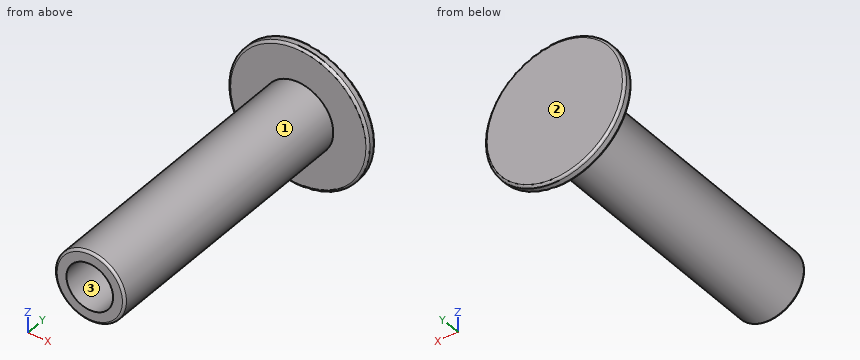
Autodesk Inventor part; units mm, degrees
ref_plane "YZ Plane" through (0, 0, 0) normal (1, 0, 0) x (0, 1, 0)
ref_plane "XZ Plane" through (0, 0, 0) normal (0, 1, 0) x (-1, 0, 0)
ref_plane "XY Plane" through (0, 0, 0) normal (0, 0, 1) x (1, 0, 0)
sketch "Boceto1" plane through (0, 0, 0) normal (0, 1, 0) x (-1, 0, 0)
  circle A0 centre (0, 0) radius 7.5
  circle A1 centre (0, 0) radius 5
  dimension "d0" = 15
  dimension "d1" = 10
extrude "Extrusión1" add sketch "Boceto1" along normal blind 60
sketch "Boceto2" plane through (0, 60, 0) normal (0, 1, 0) x (1, 0, 0)
  circle A0 centre (0, 0) radius 15
  dimension "d4" = 30
extrude "Extrusión2" add sketch "Boceto2" along normal blind 2
fillet "Empalme1" radius 0.5 1 edges at (-15, 62, 0)
fillet "Empalme2" radius 0.5 1 edges at (-15, 60, 0)
fillet "Empalme3" radius 0.5 1 edges at (7.5, 0, 0)
properties part number "contra_bici"
Build history of the part. All positions in model axes, mm. Face numbers are marked on the shaded views. Round coordinates to 2 decimals unless told otherwise and drop trailing zeros. Loops run counter-clockwise (first coordinate to the right, second up) from the corner with the lowest first, then second, coordinate; pieces in that order, holes last. Notation, with made-up numbers: (21.25, 21.25) -> (77.25, 21.25) arc R19 cw to (77.25, 34.25) -> close; hole circle Ø11 at (15.5, -24.75). An arc over 180 degrees is marked (long way). Answer in a Markdown table with one row per item.
Item 1: Drill centre lines: L1, parallel to Z at x = 0, y = 31; L2, parallel to Y at x = -14, z = 1.5; L3, parallel to Z at x = -3, y = 28. Where is each one in solid material? Low to high. Write a range as [from, to].
Answers below:
| item | result |
|---|---|
| L1 | z = [-7.5, -5], [5, 7.5] |
| L2 | y = [60, 62] |
| L3 | z = [-6.87, -4], [4, 6.87] |
Item 2: Saw through at B-B (z = 0). Write the cut outline in (x, y), and give its area (3 significant figures).
Answers below:
| item | result |
|---|---|
| outline | (-15, 60.5) arc R0.5 ccw to (-14.5, 60) -> (-7.5, 60) -> (-7.5, 0.5) arc R0.5 ccw to (-7, 0) -> (-5, 0) -> (-5, 60) -> (5, 60) -> (5, 0) -> (7, 0) arc R0.5 ccw to (7.5, 0.5) -> (7.5, 60) -> (14.5, 60) arc R0.5 ccw to (15, 60.5) -> (15, 61.5) arc R0.5 ccw to (14.5, 62) -> (-14.5, 62) arc R0.5 ccw to (-15, 61.5) -> close |
| area | 360 mm² |
Item 3: Pin check, flat tips, straight feed: pin 1 (3 mm diameter, centred on x = 4.5, y = 25, fed in from -Z); pin 2 (3 mm diameter, centred on x = -2, z = -1, fed in from -Y); pin 3 (3 mm diameter, centred on y = 34, z = -5.5, fed in from -X). Stop position of each tip, or through.
Answers below:
| item | result |
|---|---|
| pin 1 | stops at z = -6.87 |
| pin 2 | stops at y = 60 |
| pin 3 | stops at x = -6.34 |
Item 4: Saw through at A-A (x = 0). Write the cut outline in (y, z), and give its area (3 significant figures).
Answers below:
| item | result |
|---|---|
| outline | (0, -7) arc R0.5 ccw to (0.5, -7.5) -> (60, -7.5) -> (60, -14.5) arc R0.5 ccw to (60.5, -15) -> (61.5, -15) arc R0.5 ccw to (62, -14.5) -> (62, 14.5) arc R0.5 ccw to (61.5, 15) -> (60.5, 15) arc R0.5 ccw to (60, 14.5) -> (60, 7.5) -> (0.5, 7.5) arc R0.5 ccw to (0, 7) -> (0, 5) -> (60, 5) -> (60, -5) -> (0, -5) -> close |
| area | 360 mm² |
Item 5: Mould opens along Z. For the marked faces 1, 2 and 3 say: +Z half, -Z half, draft (parallel to the pull), parting line (faces both ways), or undercut.
Answers below:
| item | result |
|---|---|
| face 1 | parting line |
| face 2 | draft |
| face 3 | undercut |
Item 6: Saw through at C-C (y = 18). Write the cut outline in (x, z).
Answers below:
| item | result |
|---|---|
| outline | circle Ø15 at (0, 0); hole circle Ø10 at (0, 0) |
